CAD build for the part. Positions are in the model's coordinates, mm. A direction names the side the tool comes from. Coordinates: 2 decimals unless noted, no trailing zeros. Loops run counter-clockwise (first coordinate to the right, second up) from the corner with the lowest first, then second, coordinate; pieces in that order, holes last.
1) Saw through at A-A, the plane z = 0.75. Give the number of separate pieces and of enclosed holes in the cut face, and give its area (3 significant figures).
2) Pin check, flat tip, straight feed: pin 1 Ø2.5 at (x, y) = (9, -73.5) entering from -Z. Stop position of the tip, or through.
3) Which spindle directions (+Z, -Z, +X, -X, +Y, -Y) get a long thin tool onto all of the face, cutting with end or side? Do faces 1 (the flat face through (0, 1, 3)), 2 (the cylindrical face through (-9.293, -46.612, 1.479)), 3 (the cylindrical face through (18.06, -60.28, 1.48)). Say none if no direction does.
4) Saw through at B-B, the plane y = -55. Write the cut outline in (x, z).
5) Wall check: line 1 along Y through (x, z) = (-15, 1.05); line 2 along Y through (x, z) = (-9.5, 1.55); line 3 along Y through (x, z) = (-13, 1.5). Give the ranges that are in metal, low to high.
```python
from build123d import *

# Parameters (mm, degrees)
F0_W        = 40
F0_H        = 155
F1_DEPTH    = 3
F2_W        = 12.5
F2_H        = 13
F3_DEPTH    = 3
F4_R        = 8
F5_T1_DEPTH = 3
F6_R        = 1
F7_DEPTH    = 3


# Not quite as in the source:
# - a fillet or chamfer that OpenCascade refuses, or shapes differently, is made with other operations: its cross-section is extruded or revolved along the edge and cut away or added


with BuildPart() as f1:
    # F0 (on Top) → F1 (new body)
    with BuildSketch(Plane.XY):
        Rectangle(F0_W, F0_H)
    extrude(amount=F1_DEPTH)

    # F2 (on face) → F3 (cut, through all)
    with BuildSketch(Plane.XY.offset(3)):
        with Locations((-13.75, -51)):
            Rectangle(F2_W, F2_H)
        with Locations((13.75, -51)):
            Rectangle(F2_W, F2_H)
    extrude(amount=-F3_DEPTH, mode=Mode.SUBTRACT)

    # F4
    f4_edges = [f1.edges().sort_by_distance(p)[0] for p in [
        (-20, -44.5, 1.5),
        (20, -44.5, 1.5),
        (20, -57.5, 1.5),
        (-20, -57.5, 1.5),
        (-20, -77.5, 1.5),
        (20, -77.5, 1.5),
        (-20, 77.5, 1.5),
        (20, 77.5, 1.5),
    ]]
    fillet(f4_edges, radius=F4_R)

    # F5: fillet of radius 7 on 4 edges, made by hand

    # F5_s2 → F5_t1 (join)
    with BuildSketch(Plane.XY):
        with BuildLine():
            ThreePointArc((-13.3333333333, -44.3881063775), (-9.1536616892, -46.7717188872), (-7.5, -51.2901994578))
            Line((-7.5, -51.2901994578), (-6.8, -51.2901994578))
            Line((-6.8, -51.2901994578), (-6.8, -44.5))
            Line((-6.8, -44.5), (-7.5, -43.8))
            ThreePointArc((-7.5, -43.8), (-12, -43.8), (-13.2166666667, -43.6978970694))
            Line((-13.2166666667, -43.6978970694), (-13.3333333333, -44.3881063775))
        make_face()
        with BuildLine():
            ThreePointArc((-7.5, -50.7098005422), (-9.1536616892, -55.2282811128), (-13.3333333333, -57.6118936225))
            Line((-13.3333333333, -57.6118936225), (-13.2166666667, -58.3021029306))
            ThreePointArc((-13.2166666667, -58.3021029306), (-12, -58.2), (-7.5, -58.2))
            Line((-7.5, -58.2), (-6.8, -57.5))
            Line((-6.8, -57.5), (-6.8, -50.7098005422))
            Line((-6.8, -50.7098005422), (-7.5, -50.7098005422))
        make_face()
        with BuildLine():
            ThreePointArc((13.3333333333, -44.3881063775), (9.1536616892, -46.7717188872), (7.5, -51.2901994578))
            Line((7.5, -51.2901994578), (6.8, -51.2901994578))
            Line((6.8, -51.2901994578), (6.8, -44.5))
            Line((6.8, -44.5), (7.5, -43.8))
            ThreePointArc((7.5, -43.8), (12, -43.8), (13.2166666667, -43.6978970694))
            Line((13.2166666667, -43.6978970694), (13.3333333333, -44.3881063775))
        make_face()
        with BuildLine():
            ThreePointArc((7.5, -50.7098005422), (9.1536616892, -55.2282811128), (13.3333333333, -57.6118936225))
            Line((13.3333333333, -57.6118936225), (13.2166666667, -58.3021029306))
            ThreePointArc((13.2166666667, -58.3021029306), (12, -58.2), (7.5, -58.2))
            Line((7.5, -58.2), (6.8, -57.5))
            Line((6.8, -57.5), (6.8, -50.7098005422))
            Line((6.8, -50.7098005422), (7.5, -50.7098005422))
        make_face()
    extrude(amount=F5_T1_DEPTH)

    # F6 (on face) → F7 (cut, through all)
    with BuildSketch(Plane.XY.offset(3)):
        with Locations((-15, -73.5)):
            Circle(F6_R)
        with Locations((-9, -73.5)):
            Circle(F6_R)
        with Locations((-3, -73.5)):
            Circle(F6_R)
        with Locations((3, -73.5)):
            Circle(F6_R)
        with Locations((-15, -28.8)):
            Circle(F6_R)
        with Locations((-9, -28.8)):
            Circle(F6_R)
        with Locations((-3, -28.8)):
            Circle(F6_R)
        with Locations((3, -28.8)):
            Circle(F6_R)
        with Locations((-15, 73.5)):
            Circle(F6_R)
        with Locations((-9, 73.5)):
            Circle(F6_R)
        with Locations((-3, 73.5)):
            Circle(F6_R)
        with Locations((3, 73.5)):
            Circle(F6_R)
        with Locations((9, -73.5)):
            Circle(F6_R)
        with Locations((15, -73.5)):
            Circle(F6_R)
        with Locations((9, -28.8)):
            Circle(F6_R)
        with Locations((15, -28.8)):
            Circle(F6_R)
        with Locations((9, 73.5)):
            Circle(F6_R)
        with Locations((15, 73.5)):
            Circle(F6_R)
    extrude(amount=-F7_DEPTH, mode=Mode.SUBTRACT)


solid = f1.part
```
Data:
1. separate pieces: 1
1. enclosed holes: 18
1. area: 5,750 mm2
2. pin 1: stops at z = 0
3. face 1: +Z, +X, -X, +Y, -Y
3. face 2: +Z, -Z, -X
3. face 3: +Z, -Z, +X
4. outline: (-8.97, 0) - (8.97, 0) - (8.97, 3) - (-8.97, 3) - close
5. line 1: y = -76.92 to -74.5, -72.5 to -58.08, -43.92 to -29.8, -27.8 to 72.5, 74.5 to 76.92
5. line 2: y = -77.5 to -74.37, -72.63 to -55.61, -46.39 to -29.67, -27.93 to 72.63, 74.37 to 77.5
5. line 3: y = -77.44 to -57.55, -44.45 to 77.44
